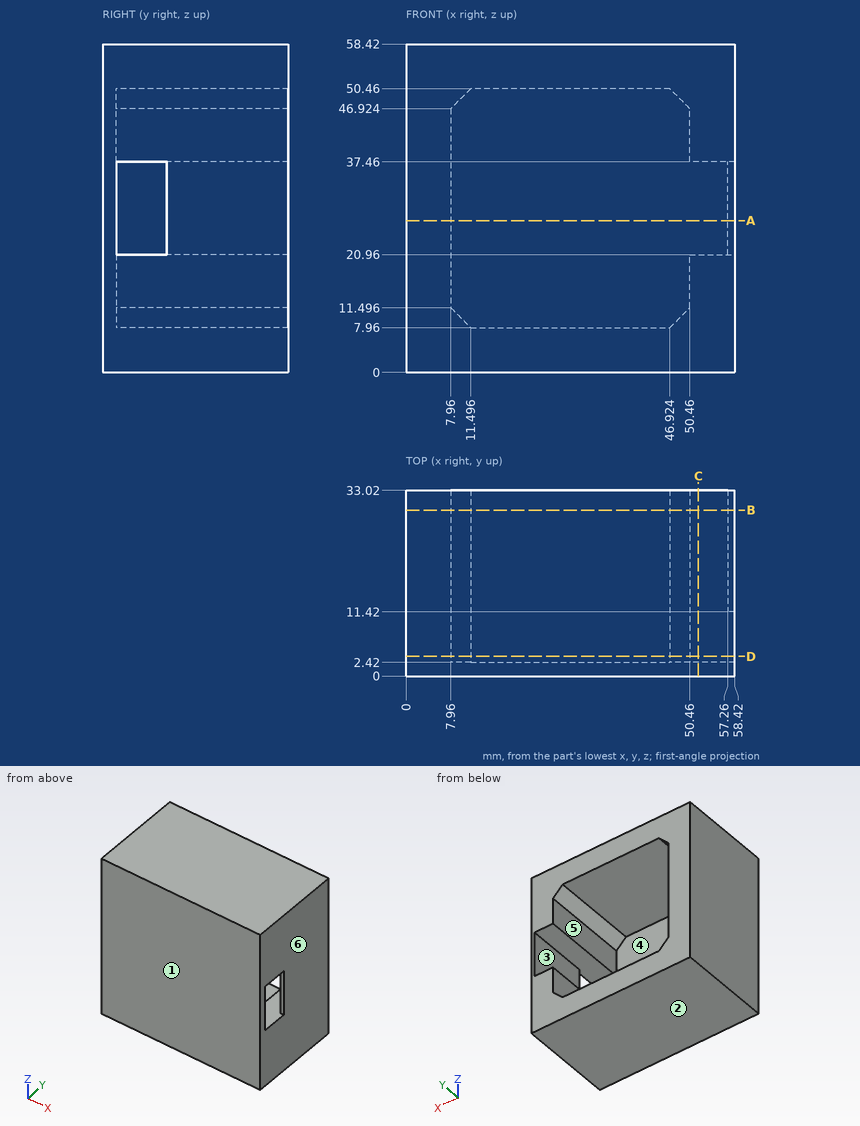
Input: dimensioned drawing with shaded views. Units: mm. Origin: part minimum x, y, z. A direction names the side the tool comes from. Coordinates: 2 decimals unless noted, no trailing zeros. Order: outer loops, then holes, each group sorted by start corner. A loop starts at its lowest first (then second) coordinate and runs counter-clockwise, first axis right, second up.
Item 1: Section query C-C (x = 52). Output: boundary loops of the cut face in (y, z), then the cut area to 3 significant figures.
Answer:
outline: (0, 0) - (33.02, 0) - (33.02, 20.96) - (2.42, 20.96) - (2.42, 37.46) - (33.02, 37.46) - (33.02, 58.42) - (0, 58.42) - close
area: 1,420 mm2
Item 2: Draft query along Z for the marked faces 1, 2, 3 and 4. Return one class per face: released by +Z, released by -Z, zero draft, split by the parting line, or undercut.
Answer:
face 1: zero draft
face 2: released by -Z
face 3: undercut
face 4: undercut
Item 3: Material intervals for line 1 along Z through (x, y) = (43.5, 28.5); line 2 along X through (y, z) = (20.5, 28), sorted ascending.
Answer:
line 1: z = 0 to 7.96, 50.46 to 58.42
line 2: x = 0 to 7.96, 57.26 to 58.42
Item 4: Section query A-A (z = 27). Output: boundary loops of the cut face in (x, y).
Answer:
outline: (0, 0) - (58.42, 0) - (58.42, 2.42) - (7.96, 2.42) - (7.96, 33.02) - (0, 33.02) - close; (57.26, 11.42) - (58.42, 11.42) - (58.42, 33.02) - (57.26, 33.02) - close
Item 5: Section query B-B (y = 29.5). Output: boundary loops of the cut face in (x, z) (1 decimal), then the cut area to 3 significant figures.
Answer:
outline: (0, 0) - (58.4, 0) - (58.4, 58.4) - (0, 58.4) - close; hole (8, 11.5) - (11.5, 8) - (46.9, 8) - (50.5, 11.5) - (50.5, 21) - (57.3, 21) - (57.3, 37.5) - (50.5, 37.5) - (50.5, 46.9) - (46.9, 50.5) - (11.5, 50.5) - (8, 46.9) - close
area: 1,520 mm2
Item 6: Access query for the marked faces 5 and 6. Directions: +Z, -Z, +X, -X, +Y, -Y. A direction counts if a zero-diameter tool reaches every point of the face in a straight line with its end or side. Return the directions, or none.
Answer:
face 5: +Y
face 6: +Z, -Z, +X, +Y, -Y
Item 7: Contact query for flat-ended pins moving along their axis: P1, Ø3, axis at x = 32, z = 34.5, coming from the -Y side; P2, Ø21, axis at x = 21.5, z = 29, coming from the +Y side. Output: stop coordinate, or through.
Answer:
P1: stops at y = 0
P2: stops at y = 2.42
Item 8: Section query D-D (y = 3.5). Output: boundary loops of the cut face in (x, z) (1 decimal).
Answer:
outline: (0, 0) - (58.4, 0) - (58.4, 21) - (50.5, 21) - (50.5, 11.5) - (46.9, 8) - (11.5, 8) - (8, 11.5) - (8, 46.9) - (11.5, 50.5) - (46.9, 50.5) - (50.5, 46.9) - (50.5, 37.5) - (58.4, 37.5) - (58.4, 58.4) - (0, 58.4) - close
